Input: part model. Units: mm. Frame: model coordinates. A direction names the side the tool comes from. Coordinates: 2 decimals unless noted, no trailing zeros. Write each loop counter-clockwise with the first axis right and the second up, starting at its lowest first coordinate (ties: lowest second). Pieces come first, ordered by that corner, then holes. Notation, with made-up numbers: M 23,46 L 81,46 A18 cw 81,63 Z; hole C 43,-0.75 d10. An arc over 180 degrees is marked long. Use one line per item in the form item = value.
from build123d import *

# Parameters (mm, degrees)
F0_W     = 50.8
F0_H     = 25.4
F1_DEPTH = 25.4
F3_DEPTH = 25.4
F5_DEPTH = 12.7
F6_W     = 50.8
F6_H     = 19.05
F7_DEPTH = 50.8


with BuildPart() as f1:
    # F0 (on Front) → F1 (new body)
    with BuildSketch(Plane.XZ):
        with Locations((25.4, 12.7)):
            Rectangle(F0_W, F0_H)
    extrude(amount=F1_DEPTH)

    # F3 (add): a face of the model
    f3_faces = [f1.faces().sort_by_distance(p)[0] for p in [
        (25.4, -12.7, 25.4),
    ]]
    extrude(f3_faces, amount=F3_DEPTH)

    # F4 (on face) → F5 (cut)
    with BuildSketch(Plane.XY.offset(50.8)):
        Polygon((50.8, -12.7), (12.7, 0), (0, 0), (0, -19.05), (19.05, -25.4), (50.8, -25.4), align=None)
    extrude(amount=-F5_DEPTH, mode=Mode.SUBTRACT)

    # F6 (on face) → F7 (cut)
    with BuildSketch(Plane(origin=(0, 0, 0), x_dir=(-1, 0, 0), z_dir=(0, 1, 0))):
        with Locations((-25.4, 9.525)):
            Rectangle(F6_W, F6_H)
    extrude(amount=-F7_DEPTH, mode=Mode.SUBTRACT)


solid = f1.part
(1) Section query C-C on x = 26.5. Return the cut outline in (y, z), plus the area to 3 significant figures.
Computed:
outline = M -25.4,19.05 L 0,19.05 L 0,50.8 L -4.6,50.8 L -4.6,38.1 L -25.4,38.1 Z
area = 542 mm^2
(2) Section query A-A on z = 45.5. Return the cut outline in (x, y).
Computed:
outline = M 0,-25.4 L 19.05,-25.4 L 0,-19.05 Z; M 12.7,0 L 50.8,-12.7 L 50.8,0 Z
(3) First-contact query: pin 1 Ø8 at (y, z) = (-6.5, 26) entering from -X; pin 2 Ø4 at (x, y) = (12.5, -8) entering from +Z. Flat tips, straight axial feed; report the tip coordinate or a pass-through.
Computed:
pin_1 = 0
pin_2 = 38.1
(4) Section query D-D on y = -17. Return the cut outline in (x, z).
Computed:
outline = M 0,19.05 L 50.8,19.05 L 50.8,38.1 L 0,38.1 Z
(5) Line query: probe 1 along Z at (x, y) = (14, -21.25); probe 2 along Y at (x, z) = (46, 47); probe 3 along Y at (x, z) = (34, 46). Output: solid intervals per line, ascending.
Computed:
probe_1 = 19.05 to 38.1
probe_2 = -11.1 to 0
probe_3 = -7.1 to 0
(6) Section query B-B on y = -8.75. Return the cut outline in (x, z).
Computed:
outline = M 0,19.05 L 50.8,19.05 L 50.8,50.8 L 38.95,50.8 L 38.95,38.1 L 0,38.1 Z
(7) Set-up query: faces 1 (the flat face through (5, -24, 50.8)), 2 (the flat face through (25, -15, 38.1)), 3 (the flat face through (9.39, -22.18, 44.54)). Return all of +Z, -Z, +X, -X, +Y, -Y with unobstructed straight access to the full face (end or side cutting, diameter ignored); none if empty.
Computed:
face_1 = +Z, +X, -X, +Y, -Y
face_2 = +Z
face_3 = +Z, +X
